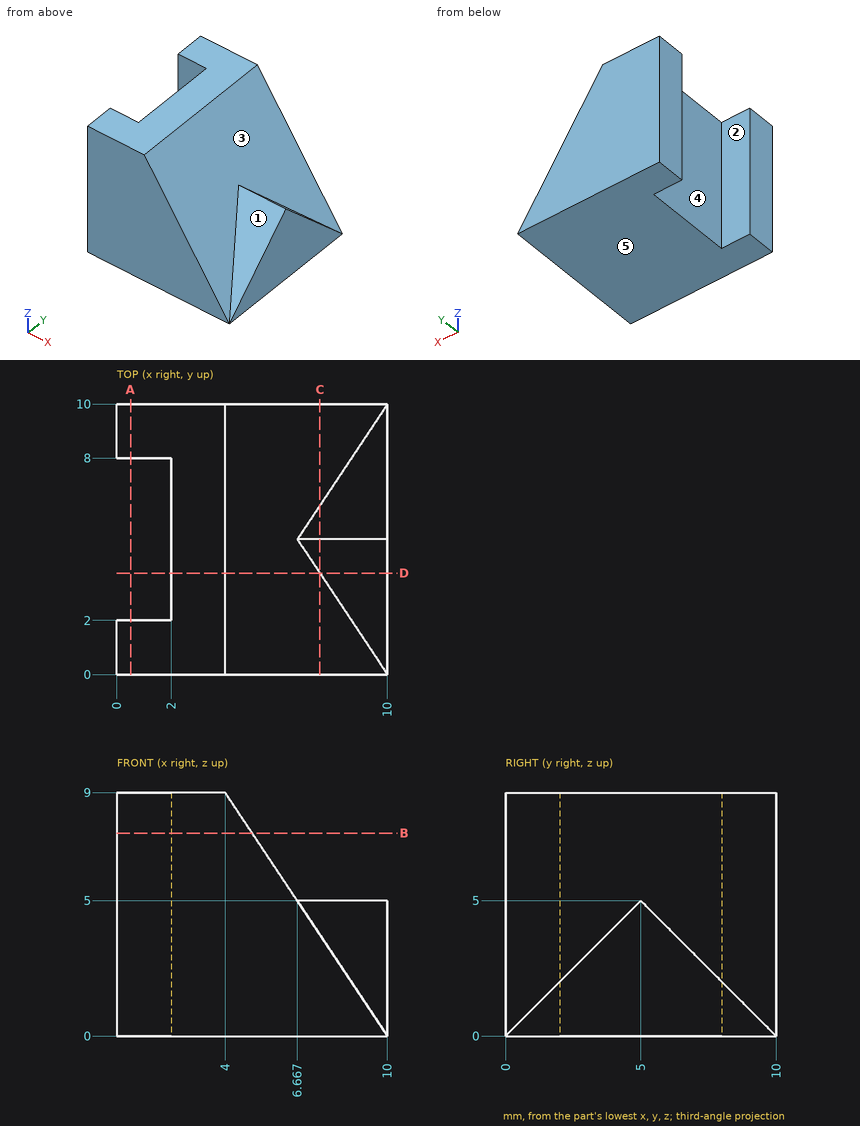
Input: dimensioned drawing with shaded views. Units: mm. Origin: part minimum x, y, z. A direction names the side the tool comes from. Round coordinates to 2 decimals unless told otherwise and drop trailing zeros. Order: outer loops, then holes, each group sorted by start corner. A loop starts at its lowest first (then second) coordinate and runs counter-clockwise, first axis right, second up.
Q1. Section B-B, the plane z = 7.5. Output: boundary loops of the cut face in (x, y), and give its area (3 significant figures).
Result sheet:
outline: (0, 0) - (5, 0) - (5, 10) - (0, 10) - (0, 8) - (2, 8) - (2, 2) - (0, 2) - close
area: 38.0 mm2
Q2. Pin query (flat end, axial travel): pin 1 (2 mm diameter, centred on x = 7.5, z = 7, fed in from +Y). Return the tip coordinate at first contact, or that it passes through.
Result sheet:
pin 1: passes through
Q3. Material intervals for probe 1 along Y at (x, z) = (0.75, 7.5); probe 2 along X at (y, z) = (7, 2.5); probe 3 along Z at (x, y) = (9.25, 2), sorted ascending.
Result sheet:
probe 1: y = 0 to 2, 8 to 10
probe 2: x = 2 to 10
probe 3: z = 0 to 2
Q4. Section A-A, the plane x = 0.5. Output: boundary loops of the cut face in (y, z), and give its area (3 significant figures).
Result sheet:
outline: (0, 0) - (2, 0) - (2, 9) - (0, 9) - close; (8, 0) - (10, 0) - (10, 9) - (8, 9) - close
area: 36.0 mm2
Q5. Access query for the marked faces 4 and 5. Directions: +Z, -Z, +X, -X, +Y, -Y. A direction counts if a zero-diameter tool reaches every point of the face in a straight line with its end or side. Return the directions, or none.
Result sheet:
face 4: +Z, -Z, -X
face 5: -Z, +X, -X, +Y, -Y
Q6. Mould query, pull axis Y, two halves, no side actions, for the marked faces 1, 2 and 3. Classes: released by +Y, released by -Y, zero draft, split by the parting line, or undercut.
Result sheet:
face 1: released by -Y
face 2: undercut
face 3: zero draft
Q7. Section C-C, the plane x = 7.5. Output: boundary loops of the cut face in (y, z).
Result sheet:
outline: (0, 0) - (10, 0) - (10, 3.75) - (6.25, 3.75) - (5, 5) - (3.75, 3.75) - (0, 3.75) - close
Q8. Section D-D, the plane y = 3.75. Output: boundary loops of the cut face in (x, z).
Result sheet:
outline: (2, 0) - (10, 0) - (10, 3.75) - (7.5, 3.75) - (4, 9) - (2, 9) - close
